Input: part model. Units: mm. Frame: model coordinates. Coordinates: 2 decimals unless noted, no trailing zeros. Write each loop counter-clockwise with the first axis right and the second up, starting at its lowest first coordinate (ties: lowest second). Pieces come first, ordered by that corner, then holes. Notation, with made-up numbers: M 64.5,-36 L 86.5,-36 A30 cw 86.5,1 Z; hole C 59,51 d3. An arc over 180 degrees is marked long. Answer as a JSON object with one key per item and string values. Group by question number.
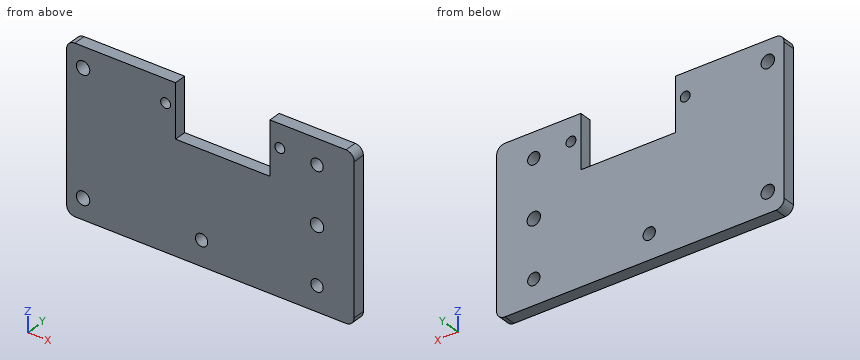
from build123d import *

# Parameters (mm, degrees)
SKETCH1_W             = 70
SKETCH1_H             = 40
BOSS_EXTRUDE1_DEPTH   = 3
F_3_0MM_DOWEL_HOLE1_D = 3
F_4_CLEARANCE_HOLE1_D = 3.2639
M2_CLEARANCE_HOLE1_D  = 2.4
SKETCH8_W             = 23
SKETCH8_H             = 13
CUT_EXTRUDE1_DEPTH    = 10
FILLET1_R             = 2


with BuildPart() as part:
    # Sketch1 → Boss-Extrude1 (new body)
    with BuildSketch(Plane(origin=(0, 0, 0), x_dir=(1, 0, 0), z_dir=(0, 1, 0))):
        Rectangle(SKETCH1_W, SKETCH1_H)
    extrude(amount=BOSS_EXTRUDE1_DEPTH)

    # Ø3.0mm Dowel Hole1 (through all)
    with Locations(Plane(origin=(0, 3, 0), x_dir=(1, 0, 0), z_dir=(0, 1, 0))):
        with Locations((-2.15, 13.9), (25.95, 13.9), (25.95, -13.9)):
            Hole(F_3_0MM_DOWEL_HOLE1_D / 2)

    # #4 Clearance Hole1 (through all)
    with Locations(Plane(origin=(0, 3, 0), x_dir=(1, 0, 0), z_dir=(0, 1, 0))):
        with Locations((-31, 15), (-31, -15), (25.95, 0)):
            Hole(F_4_CLEARANCE_HOLE1_D / 2)

    # M2 Clearance Hole1 (through all)
    with Locations(Plane(origin=(0, 3, 0), x_dir=(1, 0, 0), z_dir=(0, 1, 0))):
        with Locations((-10.9, -14.4), (16.9, -14.4)):
            Hole(M2_CLEARANCE_HOLE1_D / 2)

    # Sketch8 → Cut-Extrude1 (cut)
    with BuildSketch(Plane(origin=(0, 3, 0), x_dir=(1, 0, 0), z_dir=(0, 1, 0))):
        with Locations((3, -13.5)):
            Rectangle(SKETCH8_W, SKETCH8_H)
    extrude(amount=-CUT_EXTRUDE1_DEPTH, mode=Mode.SUBTRACT)

    # Fillet1
    fillet1_edges = [part.edges().sort_by_distance(p)[0] for p in [
        (35, 1.5, 20),
        (-35, 1.5, 20),
        (-35, 1.5, -20),
        (35, 1.5, -20),
    ]]
    fillet(fillet1_edges, radius=FILLET1_R)


solid = part.part
Q1. Section A-A, the plane x = -31. Return the cut outline in (y, z).
Q2. Section B-B, the plane z = 0. Return the cut outline in (x, y), and give its area (3 significant figures).
Q3. Pin query (flat end, axial travel): pin 1 Ø0.9 at (x, y) = (0.5, 1.5) entering from +Z. Return the tip coordinate at first contact, or that it passes through.
Q4. Section D-D, the plane x = -10.9. Return the cut outline in (y, z), and give its area (3 significant figures).
Q5. Line query: line 1 (Z direction, x = 25.95, y = 1.85); line 2 (Z direction, x = 25.5, y = 0.4); line 3 (X direction, y = 2, z = 17.5). Output: solid intervals per line, ascending. Write a range as from..to.
Q6. Section C-C, the plane y = 2.55. State how many separate pieces and enclosed holes the cut face has, and give its area (3 significant figures).
Filled in:
{
 "1": {"outline": "M 0,-20 L 3,-20 L 3,-16.63 L 0,-16.63 Z; M 0,-13.37 L 3,-13.37 L 3,13.37 L 0,13.37 Z; M 0,16.63 L 3,16.63 L 3,20 L 0,20 Z"},
 "2": {"outline": "M -35,0 L 24.32,0 L 24.32,3 L -35,3 Z; M 27.58,0 L 35,0 L 35,3 L 27.58,3 Z", "area": "200 mm^2"},
 "3": {"pin 1": "z = 7"},
 "4": {"outline": "M 0,-20 L 3,-20 L 3,13.2 L 0,13.2 Z; M 0,15.6 L 3,15.6 L 3,20 L 0,20 Z", "area": "113 mm^2"},
 "5": {"line 1": "-20..-15.4, -12.4..-1.63, 1.63..12.4, 15.4..20", "line 2": "-20..-15.33, -12.47..-1.57, 1.57..12.47, 15.33..20", "line 3": "-35..-8.5, 14.5..35"},
 "6": {"separate pieces": "1", "enclosed holes": "8", "area": "2,440 mm^2"}
}
